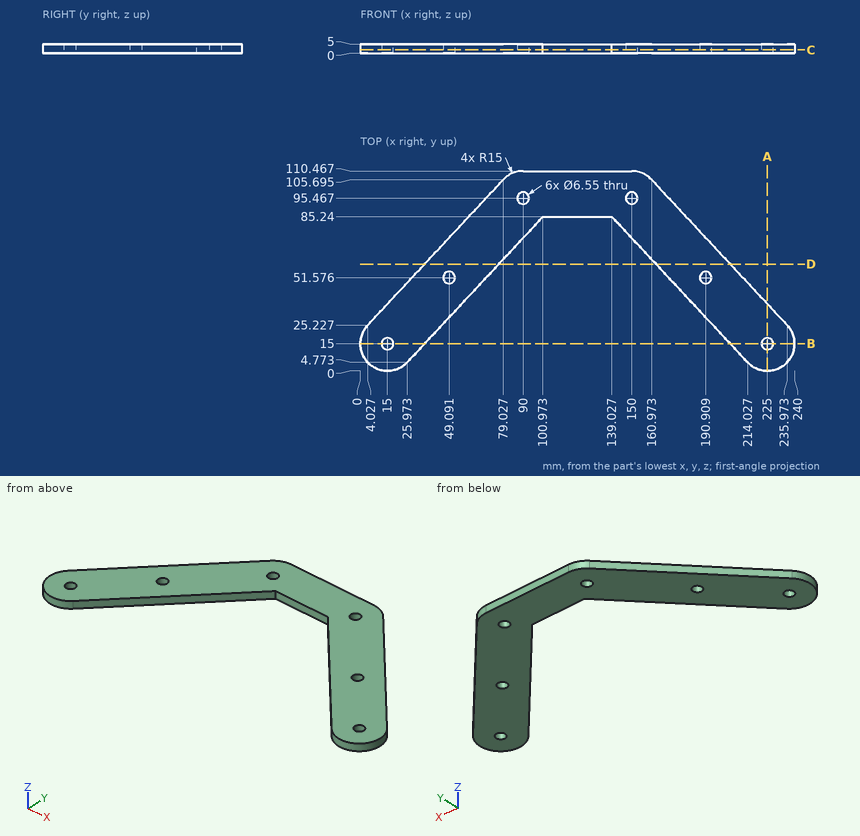
Input: dimensioned drawing with shaded views. Units: mm. Origin: part minimum x, y, z. Coordinates: 2 decimals unless noted, no trailing zeros. Order: outer loops, then holes, each group sorted by start corner. A loop starts at its lowest first (then second) coordinate and runs counter-clockwise, first axis right, second up. Notation, with made-up numbers: (64.5, 9) - (119.5, 9) arc R30 cw to (119.5, 39) - close; hole circle Ø10 at (85.5, 24). An arc over 180 degrees is marked (long way). Put each result on its own line as item: value.
1. Cut plane B-B on y = 15. Return the cut outline in (x, z) (1 decimal).
Report:
outline: (0, 0) - (11.7, 0) - (11.7, 5) - (0, 5) - close; (18.3, 0) - (35.5, 0) - (35.5, 5) - (18.3, 5) - close; (204.5, 0) - (221.7, 0) - (221.7, 5) - (204.5, 5) - close; (228.3, 0) - (240, 0) - (240, 5) - (228.3, 5) - close
2. Cut plane C-C on z = 1.75. State how many separate pieces and enclosed holes the cut face has, then the cut area to 3 significant figures.
Report:
separate pieces: 1
enclosed holes: 6
area: 8,690 mm2
3. Contact query for flat-ended pins moving along their axis: pin 1 Ø8.5 at (x, y) = (90, 95.47) entering from -Z; pin 2 Ø1.5 at (x, z) = (125.5, 3) entering from -Y; pin 3 Ø1 at (x, z) = (147.5, 4) entering from -Y; pin 4 Ø2 at (x, z) = (152, 4) entering from -Y. Output: stop coordinate, or through.
Report:
pin 1: stops at z = 0
pin 2: stops at y = 85.24
pin 3: stops at y = 75.61
pin 4: stops at y = 70.25
4. Cut plane D-D on y = 59. Return the cut outline in (x, z) (1 decimal), then the cut area to 3 significant figures.
Report:
outline: (35.5, 0) - (76.5, 0) - (76.5, 5) - (35.5, 5) - close; (163.5, 0) - (204.5, 0) - (204.5, 5) - (163.5, 5) - close
area: 410 mm2
5. Cut plane A-A on x = 225. Return the cut outline in (y, z) (1 decimal), then the cut area to 3 significant figures.
Report:
outline: (0, 0) - (11.7, 0) - (11.7, 5) - (0, 5) - close; (18.3, 0) - (37, 0) - (37, 5) - (18.3, 5) - close
area: 152 mm2
6. Line query: line 1 along X through (y, z) = (97, 2.75) (1 decimal); line 2 along X through (y, z) = (63.5, 2.9); line 3 along Y through (x, z) = (224, 3.7) (1 decimal). Output: solid intervals per line, ascending.
Report:
line 1: x = 70.9 to 87.1, 92.9 to 147.1, 152.9 to 169.1
line 2: x = 39.7 to 80.71, 159.29 to 200.3
line 3: y = 0 to 11.9, 18.1 to 38.1
